Autodesk Fusion 360 part; units mm, degrees
sketch "Sketch1" plane through (0, 0, 0) normal (0, 1, 0) x (1, 0, 0)
  line L0 (0, 0) -> (-33, 0)
  line L1 (0, 0) -> (33, 0)
  line L2 (-33, 0) -> (-38, 0)
  line L3 (33, 0) -> (38, 0)
  line L4 (-38, 0) -> (-38, -2.7218)
  line L5 (-36.2809, -6.4949) -> (-16.411, -23.773)
  line L6 (-13.1301, -25) -> (13.1301, -25)
  line L7 (38, 0) -> (38, -2.7218)
  line L8 (36.2809, -6.4949) -> (16.411, -23.773)
  arc A0 (-38, -2.7218) -> (-36.2809, -6.4949) centre (-33, -2.7218) ccw
  arc A1 (36.2809, -6.4949) -> (38, -2.7218) centre (33, -2.7218) ccw
  arc A2 (13.1301, -25) -> (16.411, -23.773) centre (13.1301, -20) ccw
  arc A3 (-16.411, -23.773) -> (-13.1301, -25) centre (-13.1301, -20) ccw
  line L9 (0, -4) -> (27.7062, -4)
  line L10 (33, -4) -> (33.0541, -4)
  line L11 (29.0185, -7.5092) -> (13.7863, -20.7546)
  arc A4 (13.1301, -21) -> (13.7863, -20.7546) centre (13.1301, -20) ccw
  line L12 (-13.1301, -21) -> (13.1301, -21)
  arc A5 (-13.7863, -20.7546) -> (-13.1301, -21) centre (-13.1301, -20) ccw
  line L13 (-29.0185, -7.5092) -> (-13.7863, -20.7546)
  line L14 (-33, -4) -> (-33.0541, -4)
  line L15 (0, -4) -> (-27.7062, -4)
  arc A6 (-27.7062, -4) -> (-29.0185, -7.5092) centre (-27.7062, -6) ccw
  arc A7 (29.0185, -7.5092) -> (27.7062, -4) centre (27.7062, -6) ccw
  dimension "d2" = 5
  dimension "d3" = 2
  dimension "d4" = 2
extrude "Extrude1" add sketch "Sketch1" along normal blind 9
sketch "Sketch2" plane through (0, 0, 0) normal (0, 0, -1) x (-1, 0, 0)
  line L0 (-38, 0) -> (38, 0)
  line L1 (38, 0) -> (38, 9)
  line L2 (38, 9) -> (-38, 9)
  line L3 (-38, 9) -> (-38, 0)
  line L4 (0, 0) -> (0, 9)
  line L5 (0, 4.5) -> (-33, 4.5)
  line L6 (0, 4.5) -> (33, 4.5)
  dimension "d7" = 33
  dimension "d8" = 33
hole "Hole1" at (33, 4.5, 0) at (-33, 4.5, 0) direction (0, 0, 1) diameter 3 depth 122 tip angle 180
sketch "Sketch3" plane through (0, 0, 25) normal (0, 0, 1) x (1, 0, 0)
  line L0 (-13.1301, 0) -> (13.1301, 0)
  line L1 (13.1301, 0) -> (13.1301, 9)
  line L2 (13.1301, 9) -> (-13.1301, 9)
  line L3 (-13.1301, 9) -> (-13.1301, 0)
  line L4 (0, 0) -> (0, 9)
  line L5 (0, 4.5) -> (-33, 4.5)
  line L6 (0, 4.5) -> (33, 4.5)
  dimension "d12" = 33
  dimension "d13" = 33
hole "Hole2" at (33, 4.5, 25) at (-33, 4.5, 25) direction (0, 0, -1) diameter 5 depth 20 tip angle 180
sketch "Sketch4" plane through (0, 0, 25) normal (0, 0, 1) x (1, 0, 0)
  line L0 (-13.1301, 0) -> (13.1301, 0)
  line L1 (13.1301, 0) -> (13.1301, 9)
  line L2 (13.1301, 9) -> (-13.1301, 9)
  line L3 (-13.1301, 9) -> (-13.1301, 0)
  line L4 (0, 4.5) -> (-9, 4.5)
  line L5 (-9, 4.5) -> (9, 4.5)
  curve L6
  curve L7
  curve L8
  curve L9
  curve L10
  curve L11
  dimension "d20" = 4.5
  dimension "d21" = 9
  dimension "d22" = 9
hole "Hole4" at (9, 4.5, 21) at (-9, 4.5, 21) direction (0, 0, 1) diameter 5 depth 1.5 tip angle 180
hole "Hole3" at (-9, 4.5, 25) at (9, 4.5, 25) direction (0, 0, -1) diameter 3 depth 20 tip angle 180
Part model, mm, in its own coordinate system. A direction names the side the tool comes from. Coordinates: 2 decimals unless noted, no trailing zeros. Write each loop counter-clockwise with the first axis right and the second up, starting at its lowest first coordinate (ties: lowest second). Pieces come first, ordered by that corner, then holes.
Item 1: Slice it at A-A (x = -4). Write the cut outline in (y, z), and give its area (3 significant figures).
Item 2: Probe line 1 (X direction, y = 4.5, z = 2.3); line 2 (Y direction, x = 33, z = 3.4); line 3 (Y direction, x = 9, z = 21.75). List the from-to ranges inside material, lowest first.
Item 3: Which spindle directions (+Z, -Z, +X, -X, +Y, -Y) get a long thin tool onto all of the face, cutting with end or side? Do faces 1 (the face through (0, 4, 21)), 2 (the face through (11, 6, 22)), 3 (the face through (10.464, 4.825, 23.732)). Say none if no direction does.
Item 4: Mould opens along Y. For faces 4 (the face through (-14.86, 4.44, 24.69)), 5 (the face through (-31.67, 5.19, 2.54)) say: released by +Y, released by -Y, zero draft, split by the parting line, or undercut.
Item 5: Slice it at B-B (y = 8.25). Write the cut outline in (x, z), and give its area (3 significant figures).
Item 6: Slice it at D-D (y = 5.25). Count the separate pieces of the cut face and the enclosed holes in it, and give its area (3 significant figures).
Item 7: Pin check, flat tips, straight feed: pin 1 (1.5 mm diameter, centred on x = -33, y = 4.5, fed in from +Z); pin 2 (1 mm diameter, centred on y = 7.5, z = 10.5, fed in from -X); pin 3 (1.5 mm diameter, centred on y = 3.5, z = 16.5, fed in from +X); pin 4 (2 mm diameter, centred on y = 1.5, z = 11.5, fed in from -X) (3 decimals). Stop position of each tip, or through.
Item 8: Slice it at C-C (z = 19). Write the cut outline in (x, y).
Results found:
1. outline: (0, 0) - (9, 0) - (9, 4) - (0, 4) - close; (0, 21) - (9, 21) - (9, 25) - (0, 25) - close
1. area: 72.0 mm2
2. line 1: x = -38 to -34.5, -31.5 to 31.5, 34.5 to 38
2. line 2: y = 0 to 3, 6 to 9
2. line 3: y = 0 to 2, 7 to 9
3. face 1: +Y, -Y
3. face 2: none
3. face 3: +Z
4. face 4: zero draft
4. face 5: undercut
5. outline: (-38, 0) - (38, 0) - (38, 2.72) arc R5 ccw to (36.28, 6.49) - (16.41, 23.77) arc R5 ccw to (13.13, 25) - (-13.13, 25) arc R5 ccw to (-16.41, 23.77) - (-36.28, 6.49) arc R5 ccw to (-38, 2.72) - close; hole (-29.02, 7.51) arc R2 ccw to (-27.71, 4) - (27.71, 4) arc R2 ccw to (29.02, 7.51) - (13.79, 20.75) arc R1 ccw to (13.13, 21) - (-13.13, 21) arc R1 ccw to (-13.79, 20.75) - close
5. area: 658 mm2
6. separate pieces: 4
6. enclosed holes: 0
6. area: 563 mm2
7. pin 1: passes through
7. pin 2: stops at x = -32.25
7. pin 3: stops at x = 25.64
7. pin 4: stops at x = -31.675
8. outline: (-21.9, 0) - (-15.8, 0) - (-15.8, 9) - (-21.9, 9) - close; (15.8, 0) - (21.9, 0) - (21.9, 9) - (15.8, 9) - close
